Part model, mm, in its own coordinate system. Face numbers are marked on the shaded views. Round coordinates to 2 decimals unless told otherwise and drop trailing zeros. Loops run counter-clockwise (first coordinate to the right, second up) from the corner with the lowest first, then second, coordinate; pieces in that order, holes last.
1) Band-saw the part on A-A, the plane z = -11. Write the cut outline in (x, y).
2) Band-saw the part on B-B, the plane x = 1.5. Write the cut outline in (y, z).
3) Drop flat-ended pins along their axis: P1, Ø5, axis at x = -11.5, z = 13, coming from the -Y side; P2, Ø8, axis at x = -18.5, z = -1, coming from the -Y side; P3, Ø9, axis at x = 0, y = 0, coming from the +Z side; P4, Ø1.5, axis at x = -56, y = -20.5, coming from the +Z side. Give the stop position or say it passes through.
4) Band-saw the part on C-C, the plane y = 3. Write the cut outline in (x, z), then the cut area to 3 significant figures.
5) Band-saw the part on D-D, the plane y = 18.5. Write the cut outline in (x, z).
6) Probe line 1 (Z direction, x = -23, y = -3); line 2 (Y direction, x = -24, z = 4.5); line 3 (Y direction, x = -50.5, z = 10). List the from-to ranges inside material, lowest first.
7) Mould opens along Z. For the marked faces 1, 2, 3 and 4 say: +Z half, -Z half, draft (parallel to the pull), parting line (faces both ways), or undercut.
from build123d import *

# Parameters (mm, degrees)
SKETCH2_R           = 7.5
BOSS_EXTRUDE2_DEPTH = 4
CUT_EXTRUDE1_DEPTH  = 67
BOSS_EXTRUDE3_DEPTH = 4


with BuildPart() as part:
    # Sketch2 → Boss-Extrude2 (new body)
    with BuildSketch(Plane.XY.offset(15)):
        with BuildLine():
            Line((-65, 30), (-65, -30))
            Line((-65, -30), (0, -25))
            ThreePointArc((0, -25), (23.150778482, 0), (0, 25))
            Line((0, 25), (-65, 30))
        make_face()
        Circle(SKETCH2_R, mode=Mode.SUBTRACT)
    extrude(amount=BOSS_EXTRUDE2_DEPTH)


with BuildPart() as body_2:
    # Mirror2: mirrored copy
    add(part.part.mirror(Plane.XY))


with BuildPart() as cut_extrude1_tool:
    # 3DSketch3 → Cut-Extrude1 (new body)
    with BuildSketch(Plane(origin=(-40.440866858, 30.316826109, 33.980744524), x_dir=(-0.63193986599376, -0.7175244265183314, 0.2929346396678423), z_dir=(0.4205608285392174, 0, 0.9072643437821234))):
        with BuildLine():
            Line((0, 0), (12.532874387, 12.166226775))
            ThreePointArc((12.532874387, 12.166226775), (12.802609816, 30.336869108), (30.973252149, 30.067133679))
            Line((30.973252149, 30.067133679), (43.506126536, 42.233360454))
            Line((43.506126536, 42.233360454), (85.796169664, 0))
            Line((85.796169664, 0), (25.881179802, -39.378555401))
            Line((25.881179802, -39.378555401), (0, 0))
        make_face()
    extrude(amount=-CUT_EXTRUDE1_DEPTH)


with BuildPart() as part_1:
    add(part.part)

    # Cut-Extrude1: cut by cut_extrude1_tool
    add(cut_extrude1_tool.part, mode=Mode.SUBTRACT)



with BuildPart() as body_2_1:
    add(body_2.part)

    # Cut-Extrude1: cut by cut_extrude1_tool
    add(cut_extrude1_tool.part, mode=Mode.SUBTRACT)


with BuildPart() as part_2:
    add(part_1.part)

    add(body_2_1.part)  # Boss-Extrude3 merges body 2
    # Sketch3 → Boss-Extrude3 (add)
    with BuildSketch(Plane(origin=(1.911764706, 24.852941176, 0), x_dir=(0.9970544855015816, -0.0766964988847369, 0), z_dir=(0.0766964988847369, 0.9970544855015816, 0))):
        Polygon((-65.249765706, 15), (-51.302234569, -15), (-18.449990724, -15), (-18.449990724, 15), align=None)
    boss_extrude3 = extrude(amount=-BOSS_EXTRUDE3_DEPTH)

    # Mirror3: Boss-Extrude3 across plane
    add(boss_extrude3.mirror(Plane.ZX))


solid = part_2.part
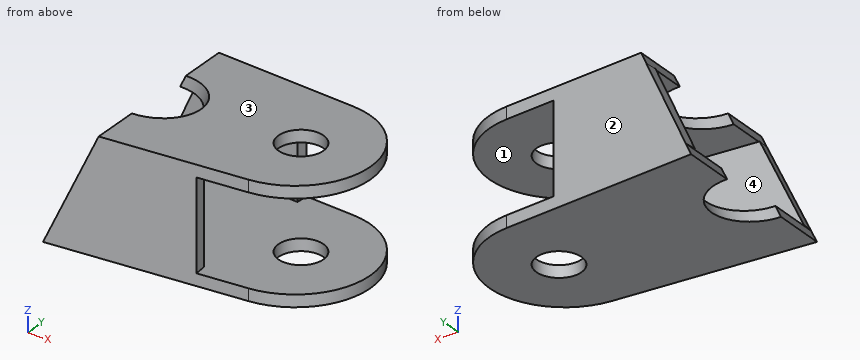
Reported:
1. outline: (-61.6, -25.73) - (-61.29, -29.71) - (-16.48, -26.27) - (-16.79, -22.28) - close; (-61.6, 25.73) - (-16.79, 22.28) - (-16.48, 26.27) - (-61.29, 29.71) - close
2. outline: (-24.84, -19) - (-7.35, -19) - (-7.35, -15) - (-24.84, -15) - close; (-24.84, 15) - (-7.35, 15) - (-7.35, 19) - (-24.84, 19) - close; (7.35, -19) - (24.84, -19) - (24.84, -15) - (7.35, -15) - close; (7.35, 15) - (24.84, 15) - (24.84, 19) - (7.35, 19) - close
3. P1: stops at y = -26
3. P2: stops at y = -26.73
3. P3: passes through
3. P4: stops at z = -15
4. outline: (-51.23, -19) - (-6.87, -19) - (-6.87, -15) - (-49.37, -15) - close; (-35.47, 15) - (-6.87, 15) - (-6.87, 19) - (-33.61, 19) - close; (6.87, -19) - (22.97, -19) - (22.97, -15) - (6.87, -15) - close; (6.87, 15) - (22.97, 15) - (22.97, 19) - (6.87, 19) - close
4. area: 413 mm2
5. outline: (-65, -19) - (15, -19) - (15, -15) - (-63.15, -15) - close; (-49.24, 15) - (15, 15) - (15, 19) - (-47.39, 19) - close
6. line 1: z = -19 to -15, 15 to 19
6. line 2: y = -26.85 to -22.83, 22.83 to 26.85
6. line 3: y = -28.88 to -24.87, 24.87 to 28.88
7. face 1: undercut
7. face 2: draft
7. face 3: +Z half
7. face 4: undercut
